Verification items for the finished model (mm, model axes). Face numbers are marked on the shaded views. Round coordinates to 2 decimals unless told otherwise and drop trailing zeros. Write each loop counter-clockwise with the first axis right and the second up, starting at its lowest first coordinate (ties: lowest second). Pieces come first, ordered by that corner, then holes. Notation, with made-up numbers: (47, 1.25) - (55, 1.25) arc R17 ccw to (55, 7.25) - close; hole circle Ø10 at (-37.75, -31). An arc over 180 degrees is marked (long way). Answer as a JSON object with one key per item and string values.
```python
from build123d import *

# Parameters (mm, degrees)
CYLINDER002_R     = 20.1
CYLINDER002_DEPTH = 30
CYLINDER001_R     = 21.5
CYLINDER001_DEPTH = 20
FILLET_R          = 1
CYLINDER_R        = 23.5
CYLINDER_DEPTH    = 2.5


with BuildPart() as cylinder002:
    # Cylinder002 → Cylinder002 (new body)
    with BuildSketch(Plane.XY.offset(2.5)):
        Circle(CYLINDER002_R)
    extrude(amount=CYLINDER002_DEPTH)


with BuildPart() as fillet_body:
    # Cylinder001 → Cylinder001 (new body)
    with BuildSketch(Plane.XY):
        Circle(CYLINDER001_R)
    extrude(amount=CYLINDER001_DEPTH)

    # Cut: cut Cylinder002
    add(cylinder002.part, mode=Mode.SUBTRACT)

    # Fillet
    fillet_edges = [fillet_body.edges().sort_by_distance(p)[0] for p in [
        (-20.1, 0, 20),
    ]]
    fillet(fillet_edges, radius=FILLET_R)


with BuildPart() as fusion:
    # Cylinder → Cylinder (new body)
    with BuildSketch(Plane.XY):
        Circle(CYLINDER_R)
    extrude(amount=CYLINDER_DEPTH)

    # Fusion: union Fillet body
    add(fillet_body.part)


solid = fusion.part
```
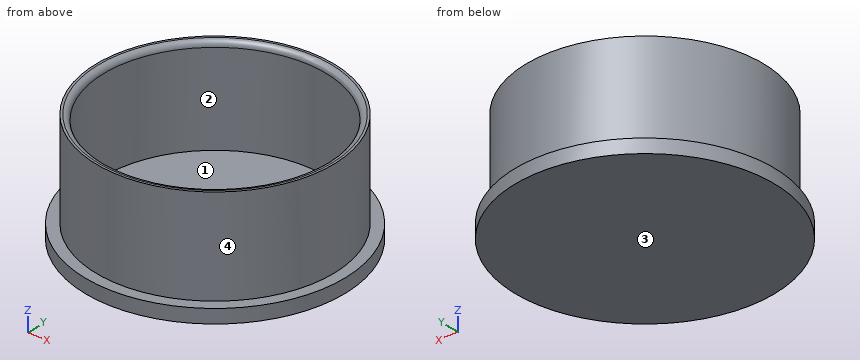
1. Cross-section at B-B (z = 11.25). Record the boundary of the cut face in (x, y), plus the area to 3 significant figures.
Completed:
{"outline": "circle Ø43 at (0, 0); hole circle Ø40.2 at (0, 0)", "area": "183 mm^2"}
2. Cross-section at A-A (y = 0). Record the boundary of the cut face in (x, z), plus the area to 3 significant figures.
Completed:
{"outline": "(-23.5, 0) - (23.5, 0) - (23.5, 2.5) - (21.5, 2.5) - (21.5, 20) - (21.1, 20) arc R1 ccw to (20.1, 19) - (20.1, 2.5) - (-20.1, 2.5) - (-20.1, 19) arc R1 ccw to (-21.1, 20) - (-21.5, 20) - (-21.5, 2.5) - (-23.5, 2.5) - close", "area": "166 mm^2"}
3. Go/stop test with flat-tipped pins: pin 1 (6 mm diameter, centred on x = 10, z = 11, fed in from +Y); pin 2 (8 mm diameter, centred on y = 3, z = 16, fed in from +X); pin 3 (8 mm diameter, centred on x = -11, y = 1, fed in from +Z). Record where each tip stops, or that it passes through.
Completed:
{"pin 1": "stops at y = 20.33", "pin 2": "stops at x = 21.5", "pin 3": "stops at z = 2.5"}
4. Material ranges on probe 1 along Y at (x, z) = (0, 7.5); probe 2 along Z at (x, y) = (-11, 13), recorded low to high. Write a range as from..to.
Completed:
{"probe 1": "y = -21.5..-20.1, 20.1..21.5", "probe 2": "z = 0..2.5"}
5. Mould release check, pull along Y, two halves, no side actions. Record for the marked faces 1, 2, 3 and 4: released by +Y, released by -Y, zero draft, split by the parting line, or undercut.
Completed:
{"face 1": "undercut", "face 2": "undercut", "face 3": "zero draft", "face 4": "split by the parting line"}
